Read the model definition and answer for the solid it produces. Units are mm, in the model's axes. Face numbers are marked on the shaded views. A direction names the side the tool comes from. Round coordinates to 2 decimals unless told otherwise and drop trailing zeros. Order: outer loops, then holes, each group sorted by start corner. A loop starts at its lowest first (then second) coordinate and runs counter-clockwise, first axis right, second up. Notation, with made-up numbers: (63.25, -4.75) -> (98.25, -4.75) arc R26 ccw to (98.25, 18.25) -> close; hole circle Ø9 at (47, 7). An arc over 180 degrees is marked (long way). One line per item, written item: value. Start each with the question number.
1. The mould has two halves that part along Z. Classify the marked faces 1, 2 and 3: released by +Z, released by -Z, zero draft, split by the parting line, or undercut.
2. Flat-ended cylindrical pins translate along their axes: pin 1 Ø3 at (x, z) = (11, -7.5) entering from +Y; pin 2 Ø4 at (x, z) = (12.5, -5) entering from -Y; pin 3 Ø6 at (y, z) = (12, -1.5) entering from +X; pin 4 Ø3 at (x, z) = (7, -5.5) entering from +Y. Find the tip coordinate at first contact, or state that the pin passes through.
3. Consider line 1 (Y direction, x = 1.35, z = -5); line 2 (X direction, y = 0.65, z = -5); line 3 (Z direction, x = 12.5, y = 1.5). Determine where each line is inside the solid, lowest interval first.
4. Section D-D (y = 9.75) is taken. Give the vertices of the cut face in (x, z), then the cut area to 3 significant figures.
5. Section C-C (z = -6) is taken. Give the vertices of the cut face in (x, y), then the cut area to 3 significant figures.
6. Section A-A (y = 12.5) is taken. Give the vertices of the cut face in (x, z).
7. For the marked faces 4, 5 and 6, determine the directions among +Z, -Z, +X, -X, +Y, -Y from which every point of the face is accessible in a straight line to the end or side of a thin tool.
from build123d import *

# Parameters (mm, degrees)
CROQUIS1_W              = 20
CROQUIS1_H              = 10
CROQUIS1_R              = 1.55
SALIENTE_EXTRUIR1_DEPTH = 3
CROQUIS2_W              = 3
CROQUIS2_H              = 10
SALIENTE_EXTRUIR2_DEPTH = 15
CROQUIS3_R              = 1.55
CORTAR_EXTRUIR1_DEPTH   = 3
CORTAR_EXTRUIR3_DEPTH   = 1
REDONDEO1_R             = 3
REDONDEO2_R             = 4
CORTAR_EXTRUIR4_DEPTH   = 1


with BuildPart() as part:
    # Croquis1 → Saliente-Extruir1 (new body)
    with BuildSketch(Plane(origin=(0, 0, 0), x_dir=(1, 0, 0), z_dir=(0, 1, 0))):
        with Locations((10, 5)):
            Rectangle(CROQUIS1_W, CROQUIS1_H)
        with Locations(Location((12.5, 5, 0), (0, 0, 270))):
            Circle(CROQUIS1_R, mode=Mode.SUBTRACT)
    extrude(amount=SALIENTE_EXTRUIR1_DEPTH)

    # Croquis2 → Saliente-Extruir2 (add)
    with BuildSketch(Plane(origin=(0, 3, 0), x_dir=(1, 0, 0), z_dir=(0, 1, 0))):
        with Locations((1.5, 5)):
            Rectangle(CROQUIS2_W, CROQUIS2_H)
    extrude(amount=SALIENTE_EXTRUIR2_DEPTH)

    # Croquis3 → Cortar-Extruir1 (cut)
    with BuildSketch(Plane.ZY):
        with Locations((-5, 12.5)):
            Circle(CROQUIS3_R)
    extrude(amount=-CORTAR_EXTRUIR1_DEPTH, mode=Mode.SUBTRACT)

    # Croquis5 → Cortar-Extruir3 (cut)
    with BuildSketch(Plane(origin=(3, 0, 0), x_dir=(0, 0, -1), z_dir=(1, 0, 0))):
        Polygon((7.9, 14.174315781), (5, 15.848631561), (2.1, 14.174315781), (2.1, 10.825684219), (5, 9.151368439), (7.9, 10.825684219), align=None)
    extrude(amount=-CORTAR_EXTRUIR3_DEPTH, mode=Mode.SUBTRACT)

    # Redondeo1
    redondeo1_edges = [part.edges().sort_by_distance(p)[0] for p in [
        (1.5, 18, 0),
        (1.5, 18, -10),
        (20, 1.5, -10),
        (20, 1.5, 0),
    ]]
    fillet(redondeo1_edges, radius=REDONDEO1_R)

    # Redondeo2
    redondeo2_edges = [part.edges().sort_by_distance(p)[0] for p in [
        (3, 3, -5),
    ]]
    fillet(redondeo2_edges, radius=REDONDEO2_R)

    # Croquis6 → Cortar-Extruir4 (cut)
    with BuildSketch(Plane(origin=(0, 3, 0), x_dir=(1, 0, 0), z_dir=(0, 1, 0))):
        Polygon((14.174315781, 7.9), (10.825684219, 7.9), (9.151368439, 5), (10.825684219, 2.1), (14.174315781, 2.1), (15.848631561, 5), align=None)
    extrude(amount=-CORTAR_EXTRUIR4_DEPTH, mode=Mode.SUBTRACT)


solid = part.part
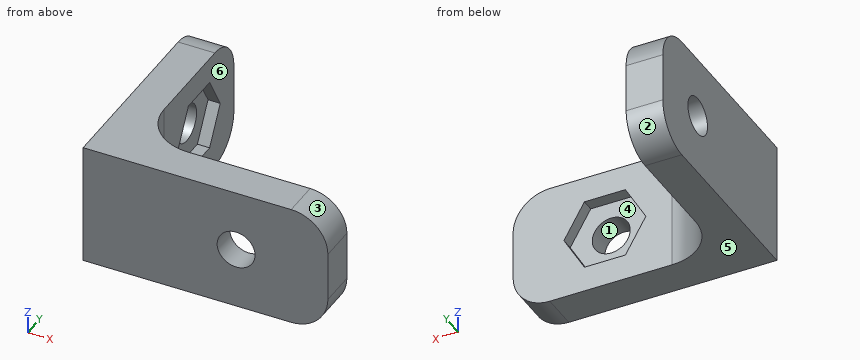
Answer:
1. face 1: undercut
1. face 2: released by -Z
1. face 3: released by +Z
2. pin 1: y = 3
2. pin 2: y = 0
2. pin 3: x = 3
2. pin 4: y = 3.29
3. line 1: 0 to 10.95, 14.05 to 18
3. line 2: 0 to 10.95, 14.05 to 20
3. line 3: -10 to -6.55, -3.45 to 0
4. outline: (0, -10) -> (3, -10) -> (3, -6.04) -> (2, -6.04) -> (2, -3.96) -> (3, -3.96) -> (3, 0) -> (0, 0) -> close
4. area: 27.9 mm^2
5. outline: (0, 0) -> (11.32, 0) -> (11.32, 2) -> (9.73, 2) -> (9.73, 3) -> (7, 3) arc R4 cw to (3, 7) -> (3, 9.73) -> (2, 9.73) -> (2, 11.32) -> (0, 11.32) -> close; (0, 13.68) -> (2, 13.68) -> (2, 15.27) -> (3, 15.27) -> (3, 18) -> (0, 18) -> close; (13.68, 0) -> (20, 0) -> (20, 3) -> (15.27, 3) -> (15.27, 2) -> (13.68, 2) -> close
5. area: 87.9 mm^2
6. outline: (0, -10) -> (3, -10) -> (3, -7.9) -> (2, -7.9) -> (2, -6.55) -> (0, -6.55) -> close; (0, -3.45) -> (2, -3.45) -> (2, -2.1) -> (3, -2.1) -> (3, 0) -> (0, 0) -> close
7. face 4: +Y
7. face 5: -Z, +X, -X, +Y, -Y
7. face 6: +Z, -Z, +X, +Y
